```python
from build123d import *

# Parameters (mm, degrees)
ESQUISSE1_R                  = 1.65
BOSS_EXTRU_1_DEPTH           = 28
ENL_V_START                  = -2.4
ESQUISSE6_R                  = 2.9
ENL_V_MAT_EXTRU_3_DEPTH      = 33.885060109
ESQUISSE7_R                  = 1.55
ENL_V_MAT_EXTRU_4_DEPTH      = 3.9
ENL_V_MAT_EXTRU_5_DEPTH      = 35.618575031
ENL_V_MAT_EXTRU_5_DEPTH_BACK = 10
ESQUISSE8_R                  = 1.2
BOSS_EXTRU_6_START           = -17
ESQUISSE10_R                 = 1.65
BOSS_EXTRU_6_DEPTH           = 6
ESQUISSE11_R                 = 1.65
ENL_V_MAT_EXTRU_6_DEPTH      = 10
ENL_V_START_2                = -10
ESQUISSE12_R                 = 1.65
ENL_V_MAT_EXTRU_7_DEPTH      = 10


with BuildPart() as part:
    # Esquisse1 → Boss.-Extru.1 (new body)
    with BuildSketch(Plane.XY):
        with BuildLine():
            Line((0, 14), (14, 4.279909917))
            Line((14, 4.279909917), (14, 2.279909917))
            Line((14, 2.279909917), (9.787977869, 2.279909917))
            ThreePointArc((9.787977869, 2.279909917), (-9.932192744, -1.534290483), (10.019692636, 0.779909917))
            Line((10.019692636, 0.779909917), (14, 0.779909917))
            Line((14, 0.779909917), (14, -14))
            Line((14, -14), (-14, -14))
            Line((-14, -14), (-14, 14))
            Line((-14, 14), (0, 14))
        make_face()
        with Locations((-11, 11)):
            Circle(ESQUISSE1_R, mode=Mode.SUBTRACT)
        with Locations(Location((-11, -11, 0), (0, 0, 180))):
            Circle(ESQUISSE1_R, mode=Mode.SUBTRACT)
        with Locations((11, -11)):
            Circle(ESQUISSE1_R, mode=Mode.SUBTRACT)
    extrude(amount=BOSS_EXTRU_1_DEPTH)

    # Esquisse6 → Enlèv. mat.-Extru.3 (cut, through all)
    with BuildSketch(Plane(origin=(0, 2.279909917, 0), x_dir=(-1, 0, 0), z_dir=(0, -1, 0)).offset(ENL_V_START)):
        with Locations((-11.8, -9)):
            Circle(ESQUISSE6_R)
        with Locations((-11.8, -19)):
            Circle(ESQUISSE6_R)
    extrude(amount=-ENL_V_MAT_EXTRU_3_DEPTH, mode=Mode.SUBTRACT)

    # Esquisse7 → Enlèv. mat.-Extru.4 (cut)
    with BuildSketch(Plane(origin=(0, 4.679909917, 0), x_dir=(1, 0, 0), z_dir=(0, 1, 0))):
        with Locations(Location((11.8, -9, 0), (0, 0, 270))):
            Circle(ESQUISSE7_R)
        with Locations(Location((11.8, -19, 0), (0, 0, 270))):
            Circle(ESQUISSE7_R)
    extrude(amount=-ENL_V_MAT_EXTRU_4_DEPTH, mode=Mode.SUBTRACT)

    # Esquisse8 → Enlèv. mat.-Extru.5 (cut, two sides: drawn at the far end of the back side and taken through both)
    with BuildSketch(Plane(origin=(0, 0.779909917, 0), x_dir=(1, 0, 0), z_dir=(0, 1, 0)).offset(-ENL_V_MAT_EXTRU_5_DEPTH_BACK)):
        with Locations((11.8, -9)):
            Circle(ESQUISSE8_R)
        with Locations((11.8, -19)):
            Circle(ESQUISSE8_R)
    extrude(amount=ENL_V_MAT_EXTRU_5_DEPTH + ENL_V_MAT_EXTRU_5_DEPTH_BACK, mode=Mode.SUBTRACT)

    # Esquisse10 → Boss.-Extru.6 (add)
    with BuildSketch(Plane.XY.offset(28).offset(BOSS_EXTRU_6_START)):
        with Locations(Location((-11, -11, 0), (0, 0, 180))):
            Circle(ESQUISSE10_R)
        with Locations((11, -11)):
            Circle(ESQUISSE10_R)
        with Locations((-11, 11)):
            Circle(ESQUISSE10_R)
    extrude(amount=BOSS_EXTRU_6_DEPTH)

    # Esquisse11 → Enlèv. mat.-Extru.6 (cut)
    with BuildSketch(Plane(origin=(0, -14, 0), x_dir=(1, 0, 0), z_dir=(0, 1, 0))):
        with Locations(Location((-11, -14, 0), (0, 0, 270))):
            Circle(ESQUISSE11_R)
        with Locations(Location((11, -14, 0), (0, 0, 90))):
            Circle(ESQUISSE11_R)
    extrude(amount=ENL_V_MAT_EXTRU_6_DEPTH, mode=Mode.SUBTRACT)

    # Esquisse12 → Enlèv. mat.-Extru.7 (cut)
    with BuildSketch(Plane(origin=(0, 14, 0), x_dir=(1, 0, 0), z_dir=(0, 1, 0)).offset(ENL_V_START_2)):
        with Locations(Location((-11, -14, 0), (0, 0, 270))):
            Circle(ESQUISSE12_R)
    extrude(amount=ENL_V_MAT_EXTRU_7_DEPTH, mode=Mode.SUBTRACT)


solid = part.part
```
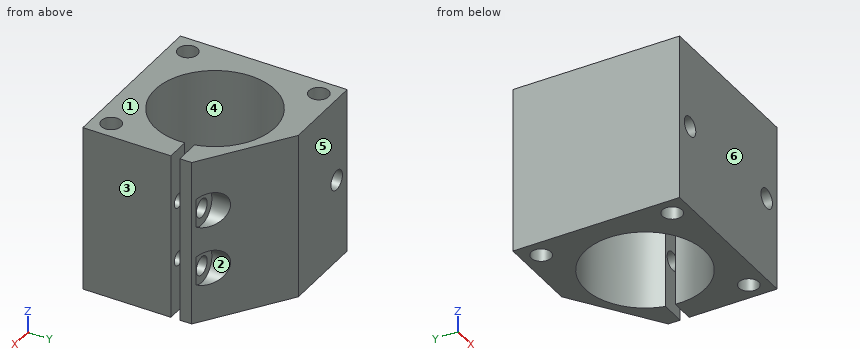
Part model, mm, in its own coordinate system. Face numbers are marked on the shaded views. A direction names the side the tool comes from. Round coordinates to 2 decimals unless told otherwise and drop trailing zeros. Loops run counter-clockwise (first coordinate to the right, second up) from the corner with the lowest first, then second, coordinate; pieces in that order, holes last.
1. Slice it at D-D (y = 7.25). Give the cut face in (x, z).
Solutions:
outline: (-14, 0) - (-6.96, 0) - (-6.96, 28) - (-14, 28) - close; (6.96, 0) - (9.72, 0) - (9.72, 6.98) arc R2.9 cw to (9.72, 11.02) - (9.72, 16.98) arc R2.9 cw to (9.72, 21.02) - (9.72, 28) - (6.96, 28) - close; hole circle Ø3.3 at (-11, 14)
2. Slice it at C-C (z = 5.25). Give the cut face in (x, y).
Solutions:
outline: (-14, -14) - (14, -14) - (14, 0.78) - (10.02, 0.78) arc R10.05 cw (long way) to (9.79, 2.28) - (14, 2.28) - (14, 4.28) - (0, 14) - (-14, 14) - close; hole circle Ø3.3 at (-11, -11); hole circle Ø3.3 at (-11, 11); hole circle Ø3.3 at (11, -11)
3. Two-plate mould, pull along Y, no slides. Class the marked faces 3, 4, 5 and 6: pulls with the +Y half, pulls with the -Y half, needs draft (parallel to the pull), parting line crosses it, or undercut.
Solutions:
face 3: needs draft
face 4: undercut
face 5: pulls with the +Y half
face 6: pulls with the -Y half
4. 3-axis set-ups, long thin cutter, end or side, ignore diameter. For the marked faces 1 and 2: which of +Z, -Z, +X, -X, +Y, -Y reach the whole face in a straight line?
Solutions:
face 1: +Z, +X, -X, +Y, -Y
face 2: +Y
5. Slice it at A-A (y = 0). Give the cut face in (x, z), and give its area (3 significant figures).
Solutions:
outline: (-14, 0) - (-10.05, 0) - (-10.05, 28) - (-14, 28) - close; (10.05, 0) - (14, 0) - (14, 28) - (10.05, 28) - close; hole circle Ø2.4 at (11.8, 9); hole circle Ø2.4 at (11.8, 19)
area: 212 mm2
6. Drill centre lines: line 1 along Z through (x, y) = (11.8, 5.5); line 2 along X through (y, z) = (-7.75, 19); line 3 along X through (y, z) = (-11.5, 8). Where is each one in solid material? Low to high.
Solutions:
line 1: z = 0 to 6.1, 11.9 to 16.1, 21.9 to 28
line 2: x = -14 to -6.4, 6.4 to 10.6, 13 to 14
line 3: x = -14 to -12.57, -9.43 to 9.43, 12.57 to 14
7. Flat gauge pins, fed straight in: pin 1 (1 mm diameter, centred on y = 6.5, z = 4.5, fed in from +X); pin 2 (0.7 mm diameter, centred on x = 11.5, z = 19.5, fed in from +Y); pin 3 (2 mm diameter, centred on x = 12, z = 16, fed in from +Y). Where does each tip first touch, or does it go through?
Solutions:
pin 1: stops at x = 11.52
pin 2: stops at y = -9.22
pin 3: stops at y = 6.36
8. Slice it at B-B (x = -11). Give the cut face in (y, z).
Solutions:
outline: (-14, 0) - (-12.65, 0) - (-12.65, 11) - (-9.35, 11) - (-9.35, 0) - (9.35, 0) - (9.35, 11) - (12.65, 11) - (12.65, 0) - (14, 0) - (14, 12.35) - (4, 12.35) - (4, 15.65) - (14, 15.65) - (14, 28) - (12.65, 28) - (12.65, 17) - (9.35, 17) - (9.35, 28) - (-9.35, 28) - (-9.35, 17) - (-12.65, 17) - (-12.65, 28) - (-14, 28) - (-14, 15.65) - (-4, 15.65) - (-4, 12.35) - (-14, 12.35) - close
